Input: part model. Units: mm. Frame: model coordinates. A direction names the side the tool comes from. Round coordinates to 2 decimals unless told otherwise and drop trailing zeros. Loops run counter-clockwise (first coordinate to the right, second up) from the corner with the lowest first, then second, coordinate; pieces in that order, holes last. Notation, with made-up numbers: M -5.75,6.25 L 16.25,6.25 A21 ccw 16.25,44.25 Z; hole C -34.75,75 d10. An arc over 180 degrees is marked long. Return JSON: item names as keys, results as strings. Group by question number.
1) Contact query for flat-ended pins moving along their axis: P1, Ø12, axis at x = 14, z = 33.5, coming from the +Y side; P2, Ø1.5, axis at x = -5, y = -7, coming from the +Z side; P3, Ø6, axis at x = 18.5, y = 8.5, coming from the -Z side. Output: stop coordinate, or through.
2) Section A-A (y = 0). Output: boundary loops of the cut face in (x, z), plus the area to 3 significant figures.
3) Material intervals for line 1 (Z direction, x = 16, y = 19); line 2 (Z direction, x = 1.5, y = -4.5), sorted ascending. Write a range as from..to.
4) Access query for faces 1 (the face through (-7.364, 0.324, 30.769)), 2 (the face through (-1, 22.579, 13)). Directions: +Z, -Z, +X, -X, +Y, -Y. A direction counts if a zero-diameter tool reaches every point of the face in a straight line with its end or side. Return the directions, or none.
5) Section B-B (x = 0). Output: boundary loops of the cut face in (y, z).
6) Section D-D (y = 11.5). Output: boundary loops of the cut face in (x, z), plus the area to 3 significant figures.
from build123d import *

# Parameters (mm, degrees)
F0_W     = 72.121516
F0_H     = 45.15715
F1_DEPTH = 25.4
F2_R     = 7.371014
F3_DEPTH = 14.986
F5_DEPTH = 41.656


with BuildPart() as f1:
    # F0 (on Top) → F1 (new body)
    with BuildSketch(Plane.XY):
        Rectangle(F0_W, F0_H)
    extrude(amount=F1_DEPTH)

    # F2 (on face) → F3 (join)
    with BuildSketch(Plane.XY.offset(25.4)):
        Circle(F2_R)
    extrude(amount=F3_DEPTH)

    # F4 (on face) → F5 (cut)
    with BuildSketch(Plane.XZ.offset(22.578575)):
        Polygon((10.064982, 44.364773), (-10.993307, 41.398816), (10.064982, 29.090097), align=None)
    extrude(amount=-F5_DEPTH, mode=Mode.SUBTRACT)


solid = f1.part
Returned:
{
 "1": {"P1": "passes through", "P2": "stops at z = 25.4", "P3": "stops at z = 0"},
 "2": {"outline": "M -36.06,0 L 36.06,0 L 36.06,25.4 L 7.37,25.4 L 7.37,30.66 L -7.37,39.28 L -7.37,25.4 L -36.06,25.4 Z", "area": "1,970 mm^2"},
 "3": {"line 1": "z = 0..25.4", "line 2": "z = 0..34.1"},
 "4": {"face 1": "+Z", "face 2": "+Z, -Z, +X, -X, +Y"},
 "5": {"outline": "M -22.58,0 L 22.58,0 L 22.58,25.4 L 7.37,25.4 L 7.37,34.97 L -7.37,34.97 L -7.37,25.4 L -22.58,25.4 Z"},
 "6": {"outline": "M -36.06,0 L 36.06,0 L 36.06,25.4 L -36.06,25.4 Z", "area": "1,830 mm^2"}
}
